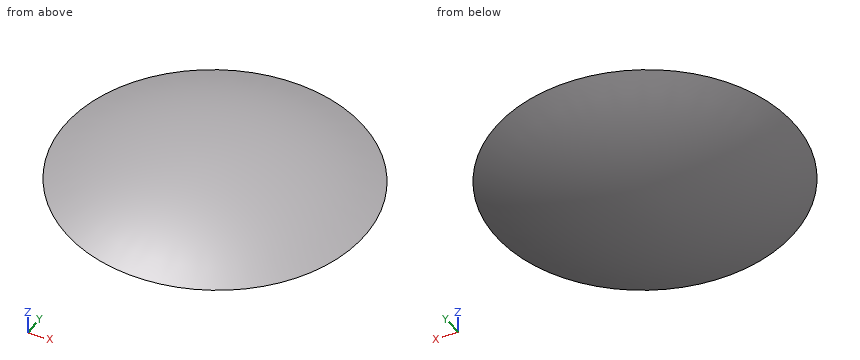
from build123d import *

# Parameters (mm, degrees)
COMMON_ROLL_ANGLE      = 1.758488
COMMON_PITCH_ANGLE     = 1.705337
COMMON_PLACEMENT_ANGLE = 1.758488


with BuildPart() as sphere001:
    # Sphere001 → Sphere001 (revolve)
    with BuildSketch(Plane(origin=(0, 0, -92), x_dir=(1, 0, 0), z_dir=(0, -1, 0))):
        with BuildLine():
            ThreePointArc((0, -51), (51, 0), (0, 51))
            Line((0, 51), (0, -51))
        make_face()
    revolve(axis=Axis((0, 0, -92), (0, 0, 1)))


with BuildPart() as common:
    # Sphere → Sphere (revolve)
    with BuildSketch(Plane.XZ):
        with BuildLine():
            ThreePointArc((0, -51), (51, 0), (0, 51))
            Line((0, 51), (0, -51))
        make_face()
    revolve(axis=Axis((0, 0, 0), (0, 0, 1)))

    # Common: intersect Sphere001
    add(sphere001.part, mode=Mode.INTERSECT)


with BuildPart() as common_1:
    # Common roll: moved
    add(common.part.rotate(Axis((0, 0, 0), (1, 0, 0)), COMMON_ROLL_ANGLE))


with BuildPart() as common_2:
    # Common pitch: moved
    add(common_1.part.rotate(Axis((0, 0, 0), (0, 1, 0)), COMMON_PITCH_ANGLE))


with BuildPart() as common_3:
    # Common placement: moved
    add(common_2.part.moved(Location((0, 0, 61))).rotate(Axis((0, 0, 61), (0, 0, 1)), COMMON_PLACEMENT_ANGLE))


solid = common_3.part
Part model, mm, in its own coordinate system. Give positions to 0.01 mm unless a question says otherwise; leave off trailing zeros. Order: outer loops, then holes, each group sorted by start corner. A loop starts at its lowest first (then second) coordinate and runs counter-clockwise, first axis right, second up. Notation, with made-up numbers: (41, 32) - (87, 32) arc R10 ccw to (87, 41) - close; hole circle Ø8 at (40.25, 86.5). An arc over 180 degrees is marked (long way). Use a Markdown table: item, result.
1) Probe L1, parallel to Z at x = -9, y = -15.5; L2, parallel to Z at x = 4, y = 17.5; L3, parallel to X at y = -0.5, z = 15.75. List the from-to ranges inside material, lowest first. Write a range as from..to.
Checked values:
| item | result |
|---|---|
| L1 | 13.25..16.31 |
| L2 | 13.26..17.42 |
| L3 | -23.14..17.5 |
2) Saw through at B-B on x = 13.5. List the corners of the cut face in (y, z).
Checked values:
| item | result |
|---|---|
| outline | (-14.81, 14.1) arc R49.18 ccw to (17.58, 15.07) arc R48.32 ccw to start |
3) Saw through at A-A on z = 11.75. List the corners of the cut face in (x, y).
Checked values:
| item | result |
|---|---|
| outline | circle Ø26.49 at (0, 0) |
4) Saw through at C-C on y = -10. List the corners of the cut face in (x, z), plus the area to 3 significant figures.
Checked values:
| item | result |
|---|---|
| outline | (-20.27, 15.28) arc R50.01 ccw to (17.43, 14.13) arc R49.38 ccw to start |
| area | 188 mm² |
5) Flat gauge pins, fed straight in: P1, Ø12, axis at x = 3, y = 15.5, coming from the -Z side; P2, Ø5, axis at x = 4, z = 17.5, coming from the +Y side; P3, Ø1, axis at x = 13, y = 8.5, coming from the +Z side. Where does each tip first touch, or does it go through?
Checked values:
| item | result |
|---|---|
| P1 | z = 10.95 |
| P2 | y = 23.05 |
| P3 | z = 17.4 |
